from build123d import *

# Parameters (mm, degrees)
F0_R     = 11
F1_DEPTH = 4
F2_R     = 1.9
F3_DEPTH = 4
F4_SIZE  = 2


with BuildPart() as f1:
    # F0 (on Top) → F1 (new body)
    with BuildSketch(Plane.XY):
        Circle(F0_R)
    extrude(amount=-F1_DEPTH)

    # F2 (on face) → F3 (join)
    with BuildSketch(Plane.XY):
        Circle(F2_R)
    extrude(amount=F3_DEPTH)

    # F4
    f4_edges = [f1.edges().sort_by_distance(p)[0] for p in [
        (-11, 0, 0),
    ]]
    chamfer(f4_edges, length=F4_SIZE)


solid = f1.part
CAD build for the part. Positions are in the model's coordinates, mm. Coordinates: 2 decimals unless noted, no trailing zeros. Loops run counter-clockwise (first coordinate to the right, second up) from the corner with the lowest first, then second, coordinate; pieces in that order, holes last. Notation, with made-up numbers: (75, -7) - (88, -7) arc R24 cw to (88, 15) - close; hole circle Ø8 at (88.25, -15). An arc over 180 degrees is marked (long way). Use one line per item in the form item = value. Start each with the question number.
1) Flat gauge pins, fed straight in: pin 1 (4 mm diameter, centred on x = -7, y = -6, fed in from +Z); pin 2 (2 mm diameter, centred on x = -2.5, z = 2, fed in from -Y); pin 3 (1.5 mm diameter, centred on x = -0.5, z = 0, fed in from +Y). Where does each tip first touch, or does it go through?
2) Band-saw the part on D-D (z = 1). Give the cut face in (x, y), and give its area (3 significant figures).
3) Band-saw the part on A-A (x = 0). Give the cut face in (y, z).
4) Band-saw the part on C-C (z = -3). Give the cut face in (x, y), and give its area (3 significant figures).
5) Two-plate mould, pull along Z, no slides. Class faces 1 (the face through (0, 0, -4)), 2 (the face through (-1.9, 0.08, 1.97)), 3 (the face through (-2.1, 0.1, 0)): +Z half, -Z half, draft (parallel to the pull), parting line (faces both ways), or undercut.
6) Drill centre lines: L1, parallel to Z at x = 2.75, y = 7; L2, parallel to Z at x = -7.5, y = -5.75; L3, parallel to X at y = -6.5, z = -2.5. Where is each one in solid material? Low to high. Write a range as from..to.
Check values:
q1.pin_1 = 0
q1.pin_2 = -1.17
q1.pin_3 = 9.74
q2.outline = circle Ø3.8 at (0, 0)
q2.area = 11.3 mm2
q3.outline = (-11, -4) - (11, -4) - (11, -2) - (9, 0) - (1.9, 0) - (1.9, 4) - (-1.9, 4) - (-1.9, 0) - (-9, 0) - (-11, -2) - close
q4.outline = circle Ø22 at (0, 0)
q4.area = 380 mm2
q5.face_1 = -Z half
q5.face_2 = draft
q5.face_3 = +Z half
q6.L1 = -4..0
q6.L2 = -4..-0.45
q6.L3 = -8.87..8.87
